Job drawing, mm, ordinate dimensions from the low corner. One solid piece. Give positions to 0.01 mm unless a question says otherwise; leave off trailing zeros. Loops run counter-clockwise (first coordinate to the right, second up) from the corner with the lowest first, then second, coordinate; pieces in that order, holes last.
Item 1: Saw through at B-B on x = 0.55. Give the cut face in (y, z).
Item 2: Probe probe 1 along Y at (x, z) = (1.2, 2.5); probe 2 along Y at (x, z) = (0.65, 2.25) (1 decimal); probe 3 along Y at (x, z) = (2, 1). List the from-to ranges inside material, lowest first.
Item 3: Drop a flat-ended pin along its axis: P1, Ø2.5, axis at y = 15.55, z = 3.15, coming from the +X side. Give the stop position or say it passes through.
Item 4: Saw through at A-A on y = 15. Give the cut face in (x, z).
Item 5: Saw through at C-C on z = 1.25. Give the cut face in (x, y), plus the area to 3 significant figures.
Item 6: Mould opens along Y. For the marked faces 1, 2, 3 and 4 say: released by +Y, released by -Y, zero draft, split by the parting line, or undercut.
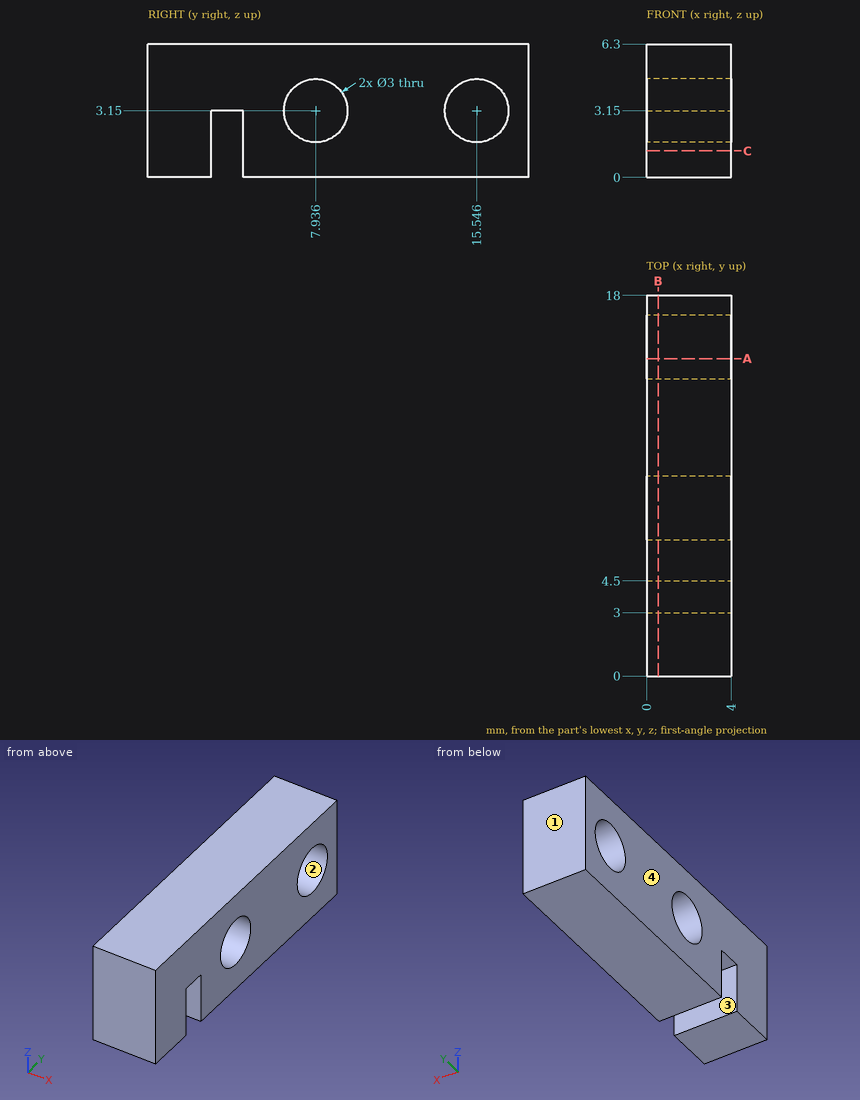
Results below:
1. outline: (0, 0) - (3, 0) - (3, 3.15) - (4.5, 3.15) - (4.5, 0) - (18, 0) - (18, 6.3) - (0, 6.3) - close; hole circle Ø3 at (7.94, 3.15); hole circle Ø3 at (15.55, 3.15)
2. probe 1: y = 0 to 3, 4.5 to 6.58, 9.29 to 14.19, 16.9 to 18
2. probe 2: y = 0 to 3, 4.5 to 6.7, 9.1 to 14.3, 16.7 to 18
2. probe 3: y = 0 to 3, 4.5 to 18
3. P1: passes through
4. outline: (0, 0) - (4, 0) - (4, 1.75) - (0, 1.75) - close; (0, 4.55) - (4, 4.55) - (4, 6.3) - (0, 6.3) - close
5. outline: (0, 0) - (4, 0) - (4, 3) - (0, 3) - close; (0, 4.5) - (4, 4.5) - (4, 18) - (0, 18) - close
5. area: 66.0 mm2
6. face 1: released by +Y
6. face 2: undercut
6. face 3: undercut
6. face 4: zero draft
